Check sheet for the modelled part. Datum: model origin and axes. Units: mm. A direction names the side the tool comes from. Round coordinates to 2 decimals unless told otherwise and drop trailing zeros. Loops run counter-clockwise (first coordinate to the right, second up) from the corner with the lowest first, then second, coordinate; pieces in that order, holes last. Notation, with made-up numbers: (9, 7) -> (22, 7) arc R16 ccw to (22, 28) -> close; hole circle Ø11 at (70.25, 85.25). An arc over 180 degrees is marked (long way). Return JSON: item names as keys, results as strings.
from build123d import *

# Parameters (mm, degrees)
F1_DEPTH      = 1
F3_R          = 0.25
F6_R          = 0.25
F7_DEPTH      = 1
F7_DEPTH_BACK = 0.25
F6_R_2        = 0.75
F8_DEPTH      = 2


with BuildPart() as f1:
    # F0 (on Top) → F1 (new body)
    with BuildSketch(Plane.XY):
        with BuildLine():
            ThreePointArc((-1.5, 0), (-1.3915219316, 0.5600595628), (-1.0817777148, 1.0391135529))
            ThreePointArc((-1.0817777148, 1.0391135529), (-1.2760507608, 1.0975033458), (-1.4776690405, 1.1198965059))
            ThreePointArc((-1.4776690405, 1.1198965059), (-1.7574719103, 0.590733833), (-1.8540965393, 0))
            Line((-1.8540965393, 0), (-1.5, 0))
        make_face()
        with BuildLine():
            ThreePointArc((-1.8540965393, 0), (-1.7574719103, 0.590733833), (-1.4776690405, 1.1198965059))
            ThreePointArc((-1.4776690405, 1.1198965059), (-2.6201191257, 0), (-1.4776690405, -1.1198965059))
            ThreePointArc((-1.4776690405, -1.1198965059), (-1.7574719103, -0.590733833), (-1.8540965393, 0))
        make_face()
        with BuildLine():
            ThreePointArc((-1.4776690405, -1.1198965059), (-1.2760507608, -1.0975033458), (-1.0817777148, -1.0391135529))
            ThreePointArc((-1.0817777148, -1.0391135529), (-1.3915219316, -0.5600595628), (-1.5, 0))
            Line((-1.5, 0), (-1.8540965393, 0))
            ThreePointArc((-1.8540965393, 0), (-1.7574719103, -0.590733833), (-1.4776690405, -1.1198965059))
        make_face()
        with BuildLine():
            ThreePointArc((1.4776690405, -1.1198965059), (1.2760507608, -1.0975033458), (1.0817777148, -1.0391135529))
            ThreePointArc((1.0817777148, -1.0391135529), (0, -1.5), (-1.0817777148, -1.0391135529))
            ThreePointArc((-1.0817777148, -1.0391135529), (-1.2760507608, -1.0975033458), (-1.4776690405, -1.1198965059))
            ThreePointArc((-1.4776690405, -1.1198965059), (0, -1.8540965393), (1.4776690405, -1.1198965059))
        make_face()
        with BuildLine():
            ThreePointArc((-1.0817777148, 1.0391135529), (0, 1.5), (1.0817777148, 1.0391135529))
            ThreePointArc((1.0817777148, 1.0391135529), (1.2760507608, 1.0975033458), (1.4776690405, 1.1198965059))
            ThreePointArc((1.4776690405, 1.1198965059), (0, 1.8540965393), (-1.4776690405, 1.1198965059))
            ThreePointArc((-1.4776690405, 1.1198965059), (-1.2760507608, 1.0975033458), (-1.0817777148, 1.0391135529))
        make_face()
        with BuildLine():
            ThreePointArc((2.6201191257, 0), (2.2841088958, 0.7999000533), (1.4776690405, 1.1198965059))
            ThreePointArc((1.4776690405, 1.1198965059), (1.7574719103, 0.590733833), (1.8540965393, 0))
            ThreePointArc((1.8540965393, 0), (1.7574719103, -0.590733833), (1.4776690405, -1.1198965059))
            ThreePointArc((1.4776690405, -1.1198965059), (2.2841088958, -0.7999000533), (2.6201191257, 0))
        make_face()
        with BuildLine():
            ThreePointArc((1.0817777148, 1.0391135529), (1.3915219316, 0.5600595628), (1.5, 0))
            ThreePointArc((1.5, 0), (1.3915219316, -0.5600595628), (1.0817777148, -1.0391135529))
            ThreePointArc((1.0817777148, -1.0391135529), (1.2760507608, -1.0975033458), (1.4776690405, -1.1198965059))
            ThreePointArc((1.4776690405, -1.1198965059), (1.7574719103, -0.590733833), (1.8540965393, 0))
            ThreePointArc((1.8540965393, 0), (1.7574719103, 0.590733833), (1.4776690405, 1.1198965059))
            ThreePointArc((1.4776690405, 1.1198965059), (1.2760507608, 1.0975033458), (1.0817777148, 1.0391135529))
        make_face()
    extrude(amount=F1_DEPTH)

    # F4: sweep along a path in F2
    with BuildLine(Plane.XZ) as f4_path:
        Line((2, 0), (2, 7))
        ThreePointArc((2, 7), (0, 9), (-2, 7))
        Line((-2, 7), (-2, 0))
    # F3 (on face) → F4 (sweep)
    with BuildSketch(Plane(origin=(0, 0, 0), x_dir=(1, 0, 0), z_dir=(0, 0, -1))):
        with Locations((2, 0)):
            Circle(F3_R)
    sweep(path=f4_path.line)

    # F6 (on offset) → F7 (join, two sides)
    with BuildSketch(Plane.XY.offset(9.25)) as f7_sk:
        Circle(F6_R)
    extrude(amount=F7_DEPTH)
    extrude(f7_sk.sketch, amount=-F7_DEPTH_BACK)

    # F6 (on offset) → F8 (join)
    with BuildSketch(Plane.XY.offset(9.25)):
        Circle(F6_R_2)
        Circle(F6_R, mode=Mode.SUBTRACT)
    extrude(amount=F8_DEPTH)


solid = f1.part
Q1. Tool access check on faces 1 (the cylindrical face through (-0.024, -1.854, 0.493)), 2 (the cylindrical face through (-0.75, 0.03, 10.24)). Record the directions out of +Z, -Z, +X, -X, +Y, -Y that give a thin tool (end or side, any length) a straight path to the whole face; none if there is none.
Results list:
{"face 1": "+Z, -Z, -Y", "face 2": "+Z"}
Q2. Section check C-C (x = -1.2). Count the separate pieces of the cut face and the enclosed holes in it, then the cut area to 3 significant figures.
Results list:
{"separate pieces": "3", "enclosed holes": "0", "area": "1.27 mm^2"}
Q3. Go/stop test with flat-tipped pins: pin 1 (1.5 mm diameter, centred on x = 1, y = 0, fed in from -Z); pin 2 (0.8 mm diameter, centred on x = -0.5, y = 0, fed in from -Z); pin 3 (2 mm diameter, centred on x = -1, z = 5.5, fed in from +Y); pin 4 (1.5 mm diameter, centred on x = -1.5, z = 8, fed in from -Y). Record where each tip stops, or that it passes through.
Results list:
{"pin 1": "z = 0", "pin 2": "z = 8.5", "pin 3": "y = 0.25", "pin 4": "y = -0.25"}
Q4. Section check A-A (x = 0). Record the boundary of the cut face in (y, z).
Results list:
{"outline": "(-1.85, 0) -> (-1.5, 0) -> (-1.5, 1) -> (-1.85, 1) -> close; (-0.75, 9.25) -> (-0.25, 9.25) -> (-0.25, 9) arc R0.25 ccw to (0.25, 9) -> (0.25, 9.25) -> (0.75, 9.25) -> (0.75, 11.25) -> (0.25, 11.25) -> (0.25, 10.25) -> (-0.25, 10.25) -> (-0.25, 11.25) -> (-0.75, 11.25) -> close; (1.5, 0) -> (1.85, 0) -> (1.85, 1) -> (1.5, 1) -> close"}
Q5. Section check B-B (z = 6.5). Record the boundary of the cut face in (x, y), then the cut area to 3 significant figures.
Results list:
{"outline": "circle Ø0.5 at (-2, 0); circle Ø0.5 at (2, 0)", "area": "0.393 mm^2"}
Q6. Material ranges on line 1 (Y direction, x = 0, z = 10.5); line 2 (Z direction, x = 1.25, y = -1.15); line 3 (Z direction, x = -0.05, y = 0.3), recorded low to high.
Results list:
{"line 1": "-0.75 to -0.25, 0.25 to 0.75", "line 2": "0 to 1", "line 3": "9.25 to 11.25"}
